from build123d import *

# Parameters (mm, degrees)
F_1_8_0_125_DIAMETER_HOLE1_D = 3.175


with BuildPart() as part:
    # Sketch1 → Revolve1 (revolve)
    with BuildSketch(Plane.XY):
        Polygon((0.150394737, -4.879473684), (-14.137105263, -4.879473684), (-14.137105263, 1.470526316), (-3.024605263, 1.470526316), (-3.024605263, 20.520526316), (0.150394737, 20.520526316), align=None)
    revolve(axis=Axis((9.675394737, 1.470526316, 0), (0, -1, 0)))

    # 1/8 (0.125) Diameter Hole1 (through all)
    with Locations(Plane(origin=(0, 1.470526316, 0), x_dir=(1, 0, 0), z_dir=(0, 1, 0))):
        with Locations((3.220899988, -17.923225088), (-9.073820881, -3.371856123), (-2.619326132, 14.551368965), (16.129889486, 17.923225088), (28.424610355, 3.371856123), (21.970115606, -14.551368965), (9.675394737, 0)):
            Hole(F_1_8_0_125_DIAMETER_HOLE1_D / 2)


solid = part.part
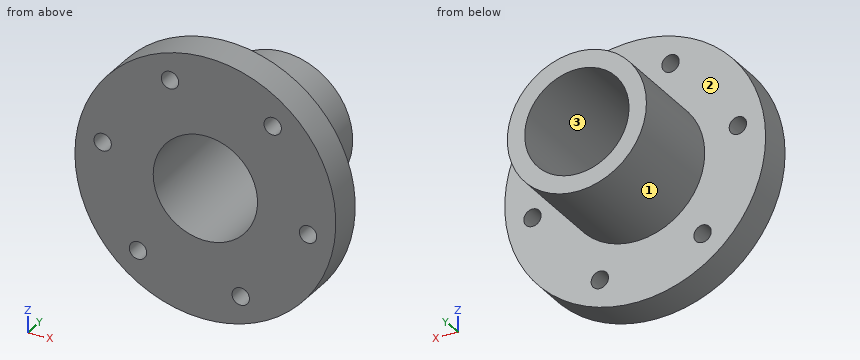
Can you work these out from the model? Positions are in its coordinate system, mm. Face numbers are marked on the shaded views. Round coordinates to 2 decimals unless told otherwise and drop trailing zeros. Write each loop counter-clockwise with the first axis right and the second up, starting at its lowest first coordinate (ties: lowest second). Pieces come first, ordered by that corner, then holes. Notation, with made-up numbers: M 11,-37.5 L 64,-37.5 A6 ccw 64,-33.5 Z; hole C 13.5,43.5 d9. An arc over 180 degrees is marked long. Use CSV: the item, a comma, the result in double quotes.
(1) Imagine slicing it at C-C (y = 0.75). Count the separate pieces of the cut face and the enclosed holes in it, plus the area to 3 significant figures.
Check values:
separate pieces,"1"
enclosed holes,"7"
area,"1,450 mm^2"
(2) I need wall thicknesses on line 1 along Y through (x, z) = (22, 8); line 2 along Z through (x, y) = (8, 6); line 3 along Z through (x, y) = (5, -0.75). Which ranges of each line are inside material? Lowest first, please.
Check values:
line 1,"-4.88 to 1.47"
line 2,"-12.59 to -9.38, 9.38 to 12.59"
line 3,"-23.35 to -8.3, 8.3 to 23.35"
(3) We'd pull the mould along X, two halves only. Please class the marked faces 1, 2 and 3: +X half, -X half, draft (parallel to the pull), parting line (faces both ways), or undercut.
Check values:
face 1,"parting line"
face 2,"draft"
face 3,"undercut"
(4) Imagine slicing it at B-B (y = 18.5). Write out the boundary of the cut face in (x, z) (3 decimals), plus the area to 3 significant figures.
Check values:
outline,"C 9.675,0 d25.4; hole C 9.675,0 d19.05"
area,"222 mm^2"
(5) I'm going to push flat-ended pins straight in: pin 1 (8 mm diameter, centred on y = 15.5, z = -2.5, fed in from +X); pin 2 (2 mm diameter, centred on y = 1.5, z = 8, fed in from +X); pin 3 (15 mm diameter, centred on x = 9.68, z = 0, fed in from -Y); pin 4 (5 mm diameter, centred on y = 15.5, z = -12.5, fed in from +X). Where does each tip first touch, or does it pass through?
Check values:
pin 1,"x = 22.38"
pin 2,"x = 32.44"
pin 3,"through"
pin 4,"x = 17.5"
(6) Imagine slicing it at A-A (z = 0). Write out the boundary of the cut face in (x, y), plus the area to 3 significant figures.
Check values:
outline,"M -14.14,-4.88 L 0.15,-4.88 L 0.15,20.52 L -3.02,20.52 L -3.02,1.47 L -14.14,1.47 Z; M 19.2,-4.88 L 33.49,-4.88 L 33.49,1.47 L 22.38,1.47 L 22.38,20.52 L 19.2,20.52 Z"
area,"302 mm^2"
